Source: three-view drawing plus pictorial views. Frame: mm from the lowest corner of the part. Give positions to 0.01 mm unless a question says otherwise; leave off trailing zeros. Order: outer loops, then holes, each group sorted by start corner. A loop starts at its lowest first (then second) coordinate and runs counter-clockwise, first axis right, second up.
1) Section B-B, the plane x = 13. Return loops of the section in (y, z) (1 decimal).
2) Draft query along X for the marked faces 1 and 2. Return one class per face: released by +X, released by -X, zero draft, split by the parting line, or undercut.
3) Section A-A, the plane x = 8. Return loops of the section in (y, z).
4) Section C-C, the plane z = 3. Return loops of the section in (x, y) (1 decimal).
5) First-contact query: P1, Ø0.5, axis at y = 5.5, z = 16.5, coming from the +X side; P2, Ø1.5, axis at x = 9, y = 4, coming from the -Z side; P3, Ø0.5, axis at y = 3.5, z = 16.5, coming from the -X side. Flat tips, straight axial feed; report the tip coordinate or a pass-through.
6) Material intervals for line 1 (Z direction, x = 8, y = 1.5); line 2 (X direction, y = 2.75, z = 5.5) (1 decimal); line 3 (X direction, y = 4.5, z = 10) (1 decimal), sorted ascending.
7) Section D-D, the plane y = 0.5. Give the number of separate pieces and of enclosed holes in the cut face.
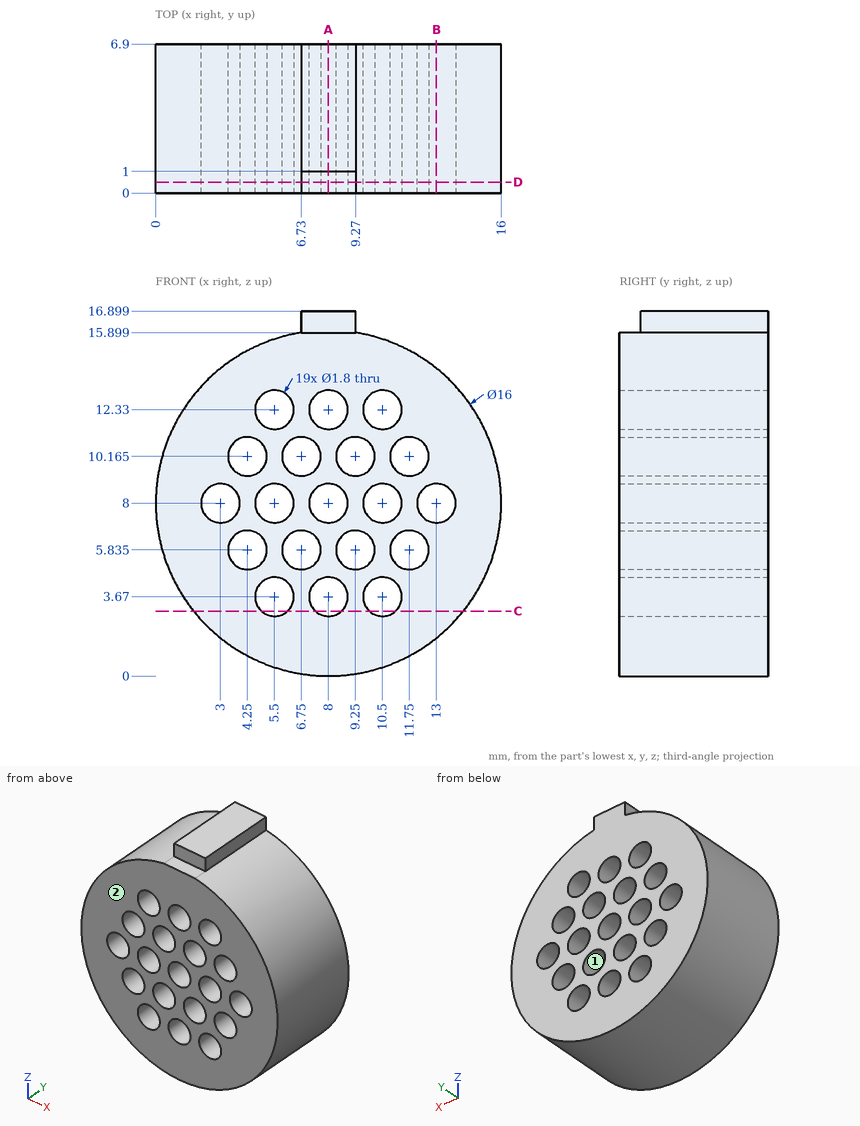
From the geometry:
1. outline: (0, 1.8) - (6.9, 1.8) - (6.9, 7.1) - (0, 7.1) - close; (0, 8.9) - (6.9, 8.9) - (6.9, 14.2) - (0, 14.2) - close
2. face 1: undercut
2. face 2: zero draft
3. outline: (0, 0) - (6.9, 0) - (6.9, 2.77) - (0, 2.77) - close; (0, 4.57) - (6.9, 4.57) - (6.9, 7.1) - (0, 7.1) - close; (0, 8.9) - (6.9, 8.9) - (6.9, 11.43) - (0, 11.43) - close; (0, 13.23) - (6.9, 13.23) - (6.9, 16.9) - (1, 16.9) - (1, 15.9) - (0, 15.9) - close
4. outline: (1.8, 0) - (4.9, 0) - (4.9, 6.9) - (1.8, 6.9) - close; (6.1, 0) - (7.4, 0) - (7.4, 6.9) - (6.1, 6.9) - close; (8.6, 0) - (9.9, 0) - (9.9, 6.9) - (8.6, 6.9) - close; (11.1, 0) - (14.2, 0) - (14.2, 6.9) - (11.1, 6.9) - close
5. P1: stops at x = 9.27
5. P2: stops at z = 0
5. P3: stops at x = 6.73
6. line 1: z = 0 to 2.77, 4.57 to 7.1, 8.9 to 11.43, 13.23 to 16.9
6. line 2: x = 0.4 to 3.4, 5.1 to 5.9, 7.6 to 8.4, 10.1 to 10.9, 12.6 to 15.6
6. line 3: x = 0.3 to 3.4, 5.1 to 5.9, 7.6 to 8.4, 10.1 to 10.9, 12.6 to 15.7
7. separate pieces: 1
7. enclosed holes: 19
